Could you check a few things on this model? Use its own coordinates, in mm. Face numbers are marked on the shaded views. Give positions to 0.01 mm unless a question says otherwise; leave off trailing zeros. Order: outer loops, then holes, each group sorted by start corner. A loop starts at its lowest first (then second) coordinate and runs counter-clockwise, first axis right, second up. Notation, with made-up numbers: (-4, 17.25) - (50, 17.25) arc R16 ccw to (50, 39.25) - close; hole circle Ø9 at (44, 0.25). An arc over 180 degrees is marked (long way). One line per question, with ' | ' between items. Start each with the question number.
1. If we mould it in two halves opening along X, with no side actions, what happens to the marked faces 1, 2 and 3? For each: released by +X, released by -X, zero draft, split by the parting line, or undercut.
2. Imagine slicing it at C-C (x = 7.25). Please give me the cut outline in (y, z), and give its area (3 significant figures).
3. Imagine slicing it at D-D (z = 5.25). Please give me the cut outline in (x, y).
4. Imagine slicing it at A-A (x = 0). Please give me the cut outline in (y, z).
5. For P1, Ø2, axis at x = 8, z = 0.5, coming from the +Y side; P2, Ø1, axis at y = -4, z = 4, coming from the -X side; P3, Ø1.5, axis at y = 5.5, z = 1.5, coming from the -X side, each with a flat end and sliding along its axis, tell me the tip position at first contact or that it passes through.
6. I need wall thicknesses on probe 1 along Y at (x, z) = (0, 1.4); probe 2 along X at (y, z) = (-0.25, 4.35); probe 3 along Y at (x, z) = (-0.75, 2.25). Which ranges of each line are inside material? Lowest first, please. Write a range as from..to.
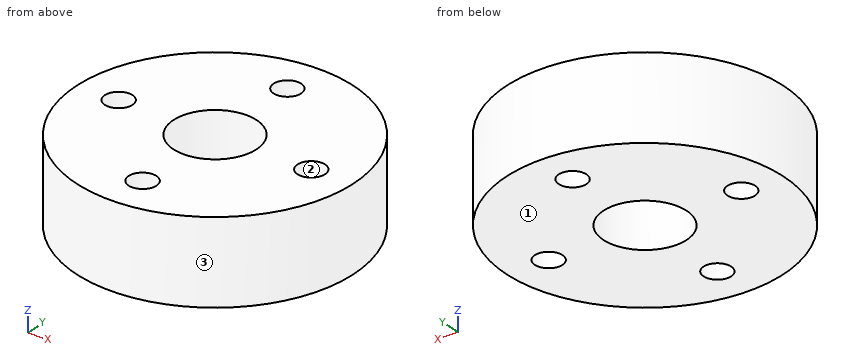
Autodesk Inventor part; units mm, degrees
ref_plane "YZ Plane" through (0, 0, 0) normal (1, 0, 0) x (0, 1, 0)
ref_plane "XZ Plane" through (0, 0, 0) normal (0, 1, 0) x (-1, 0, 0)
ref_plane "XY Plane" through (0, 0, 0) normal (0, 0, 1) x (1, 0, 0)
sketch "スケッチ1" plane through (0, 0, 0) normal (0, 0, 1) x (1, 0, 0)
  circle A0 centre (0, 0) radius 3
  circle A1 centre (0, 0) radius 10
  dimension "d0" = 6
  dimension "d1" = 20
extrude "押し出し1" add sketch "スケッチ1" along normal blind 6
sketch "スケッチ3" plane through (0, 0, 6) normal (0, 0, 1) x (1, 0, 0)
  circle A0 centre (0, 0) radius 10
  circle A1 centre (0, 0) radius 7 construction
  circle A2 centre (-7, 0) radius 1
  circle A3 centre (-4.9497, -4.9497) radius 1
  circle A4 centre (4.9497, -4.9497) radius 1
  circle A5 centre (0, -7) radius 1
  circle A6 centre (7, 0) radius 1
  circle A7 centre (4.9497, 4.9497) radius 1
  circle A8 centre (0, 7) radius 1
  circle A9 centre (-4.9497, 4.9497) radius 1
  circle A10 centre (0, 0) radius 5
  circle A11 centre (0, 0) radius 10
  circle A12 centre (0, 0) radius 7 construction
  circle A13 centre (-7, 0) radius 1
  circle A14 centre (-4.9497, -4.9497) radius 1
  circle A15 centre (4.9497, -4.9497) radius 1
  circle A16 centre (0, -7) radius 1
  circle A17 centre (7, 0) radius 1
  circle A18 centre (4.9497, 4.9497) radius 1
  circle A19 centre (0, 7) radius 1
  circle A20 centre (-4.9497, 4.9497) radius 1
  circle A21 centre (0, 0) radius 5
  dimension "d9" = 14
  dimension "d20" = 14
  dimension "d8" = 20
  dimension "d10" = 2
  dimension "d11" = 2
  dimension "d12" = 2
  dimension "d13" = 2
  dimension "d14" = 2
  dimension "d15" = 2
  dimension "d16" = 2
  dimension "d17" = 2
  dimension "d18" = 10
  dimension "d19" = 20
  dimension "d21" = 2
  dimension "d22" = 2
  dimension "d23" = 2
  dimension "d24" = 2
  dimension "d25" = 2
  dimension "d26" = 2
  dimension "d27" = 2
  dimension "d28" = 2
  dimension "d29" = 10
extrude "押し出し3" cut sketch "スケッチ3" against normal blind 10 contours A2 | A5 | A6 | A8
properties part number "Gear20"
Results found:
1) face 1: zero draft | face 2: undercut | face 3: split by the parting line
2) outline: (-6.89, 0) - (-0.97, 0) - (-0.97, 6) - (-6.89, 6) - close; (0.97, 0) - (6.89, 0) - (6.89, 6) - (0.97, 6) - close | area: 71.0 mm2
3) outline: circle Ø20 at (0, 0); hole circle Ø2 at (-7, 0); hole circle Ø6 at (0, 0); hole circle Ø2 at (0, -7); hole circle Ø2 at (0, 7); hole circle Ø2 at (7, 0)
4) outline: (-10, 0) - (-8, 0) - (-8, 6) - (-10, 6) - close; (-6, 0) - (-3, 0) - (-3, 6) - (-6, 6) - close; (3, 0) - (6, 0) - (6, 6) - (3, 6) - close; (8, 0) - (10, 0) - (10, 6) - (8, 6) - close
5) P1: stops at y = 7.14 | P2: stops at x = -9.37 | P3: stops at x = -8.8
6) probe 1: y = -10..-8, -6..-3, 3..6, 8..10 | probe 2: x = -10..-7.97, -6.03..-2.99, 2.99..6.03, 7.97..10 | probe 3: y = -9.97..-7.66, -6.34..-2.9, 2.9..6.34, 7.66..9.97
